Geometry: final body of the model. Coordinates: model frame, mm. A direction names the side the tool comes from. Give positions to 0.01 mm unless a question says otherwise; leave off trailing zeros. Write each loop counter-clockwise with the first axis right and the second up, starting at its lowest first coordinate (ties: lowest second). Pieces come first, ordered by that corner, then holes. Notation, with made-up numbers: (-19, -28.5) - (38, -28.5) arc R16 cw to (38, -3.5) - close; hole circle Ø9 at (25.5, 65). An arc over 180 degrees is marked (long way). Return JSON: item names as keys, results as strings.
from build123d import *

# Parameters (mm, degrees)
CUT_EXTRUDE1_DEPTH = 5


with BuildPart() as part:
    # Sketch1 → Revolve1 (revolve)
    with BuildSketch(Plane.XY, mode=Mode.PRIVATE) as revolve1_sk:
        with BuildLine():
            Line((12.5, 0), (0, 0))
            Line((0, 0), (0, 6.75))
            Line((0, 6.75), (5, 6.75))
            Line((5, 6.75), (5, 9.5))
            Line((5, 9.5), (8.124038405, 9.5))
            ThreePointArc((8.124038405, 9.5), (11.353424154, 5.229699797), (12.5, 0))
        make_face()
    revolve(revolve1_sk.sketch.rotate(Axis((0, 0, 0), (0, 1, 0)), 90), axis=Axis((0, 0, 0), (0, 1, 0)))

    # Sketch2 → Cut-Extrude1 (cut)
    with BuildSketch(Plane(origin=(0, 0, 0), x_dir=(1, 0, 0), z_dir=(0, 1, 0))):
        Polygon((0, 9), (2.556172718, 3.518269915), (8.559508647, 2.781152949), (4.13597434, -1.343859526), (5.290067271, -7.281152949), (0, -4.348820778), (-5.290067271, -7.281152949), (-4.13597434, -1.343859526), (-8.559508647, 2.781152949), (-2.556172718, 3.518269915), align=None)
    extrude(amount=CUT_EXTRUDE1_DEPTH, mode=Mode.SUBTRACT)


solid = part.part
Q1. Section query C-C, the plane z = 5.5. Return the cut outline in (x, y), plus the area to 3 significant figures.
Answer key:
{"outline": "(-11.22, 0) - (-4.94, 0) - (-4.94, 5) - (-2.08, 5) - (-2.08, 0) - (2.08, 0) - (2.08, 5) - (4.94, 5) - (4.94, 0) - (11.22, 0) arc R11.22 ccw to (5.98, 9.5) - (-5.98, 9.5) arc R11.22 ccw to start", "area": "155 mm^2"}
Q2. Mould query, pull axis Z, two halves, no side actions, for faces 1 (the flat face through (-4.72, 2.46, 4.35)), 2 (the flat face through (-6, 0, 0)). Classes: pulls with the +Z half, pulls with the -Z half, needs draft (parallel to the pull), parting line crosses it, or undercut.
Answer key:
{"face 1": "undercut", "face 2": "needs draft"}
Q3. Section query D-D, the plane y = 1.5. Return the cut outline in (x, z).
Answer key:
{"outline": "circle Ø24.82 at (0, 0); hole (-8.56, -2.78) - (-2.56, -3.52) - (0, -9) - (2.56, -3.52) - (8.56, -2.78) - (4.14, 1.34) - (5.29, 7.28) - (0, 4.35) - (-5.29, 7.28) - (-4.14, 1.34) - close"}
Q4. Material intervals for probe 1 along Y at (x, z) = (-3, 2); probe 2 along X at (y, z) = (8.8, 0); probe 3 along Z at (x, y) = (-3.75, 7.5), sorted ascending. Write a range as [from, to].
Answer key:
{"probe 1": "y = [5, 6.75]", "probe 2": "x = [-8.88, -5], [5, 8.88]", "probe 3": "z = [-9.27, -3.31], [3.31, 9.27]"}
Q5. Pin query (flat end, axial travel): P1, Ø3, axis at x = -0.5, z = 2.5, coming from the +Y side; P2, Ø5, axis at y = 3.5, z = 4.5, coming from the -X side; P3, Ø1.5, axis at x = -4.5, y = 1.5, coming from the -Z side. Return the tip coordinate at first contact, or that it passes through.
Answer key:
{"P1": "stops at y = 6.75", "P2": "stops at x = -12.08", "P3": "stops at z = -11.84"}
Q6. Section query B-B, the plane x = -1. Return the cut outline in (y, z).
Answer key:
{"outline": "(0, -12.46) arc R12.46 ccw to (9.5, -8.06) - (9.5, -4.9) - (6.75, -4.9) - (6.75, 4.9) - (9.5, 4.9) - (9.5, 8.06) arc R12.46 ccw to (0, 12.46) - (0, 4.9) - (5, 4.9) - (5, -6.86) - (0, -6.86) - close"}
Q7. Section query A-A, the plane y = 3. Return the cut outline in (x, z).
Answer key:
{"outline": "circle Ø24.27 at (0, 0); hole (-8.56, -2.78) - (-2.56, -3.52) - (0, -9) - (2.56, -3.52) - (8.56, -2.78) - (4.14, 1.34) - (5.29, 7.28) - (0, 4.35) - (-5.29, 7.28) - (-4.14, 1.34) - close"}
Q8. Set-up query: faces 3 (the flat face through (5.3, 9.5, -0.1)), 4 (the cylindrical face through (0, 8, 5)), 5 (the flat face through (4.705, 2.465, 4.271)). Return all of +Z, -Z, +X, -X, +Y, -Y with unobstructed straight access to the full face (end or side cutting, diameter ignored); none if empty.
Answer key:
{"face 3": "+Z, -Z, +X, -X, +Y", "face 4": "+Y", "face 5": "-Y"}
